Verification items for the finished model (mm, model axes). Coordinates: 2 decimals unless noted, no trailing zeros. Order: outer loops, then holes, each group sorted by start corner. A loop starts at its lowest first (then second) coordinate and runs counter-clockwise, first axis right, second up.
Q1. Cross-section at C-C, the plane y = 32. Record the boundary of the cut face in (x, z).
Q2. Depth check by flat-ended pin: P1, Ø4, axis at x = 9, z = 31, coming from the +Y side; P2, Ø1, axis at x = 8.5, z = 25.5, coming from the +Y side; P3, Ø5, axis at x = 10, y = 21.5, coming from the -Z side. Enter the tip coordinate at first touch or a pass-through.
Q3. Cross-section at B-B, the plane z = 28. Record the boundary of the cut face in (x, y).
Q4. Thickness scan on line 1 (Y direction, x = 3.25, z = 3); line 2 (Y direction, x = 1, z = 3.5); line 3 (Z direction, x = 9, y = 32.5). Record the ranges inside material, lowest first.
from build123d import *

# Parameters (mm, degrees)
BOSS_EXTRUDE1_DEPTH = 12.7
FILLET1_R           = 38.1
FILLET2_R           = 38.1


with BuildPart() as part:
    # Sketch1 → Boss-Extrude1 (new body)
    with BuildSketch(Plane(origin=(0, 0, 0), x_dir=(0, 0, -1), z_dir=(1, 0, 0))):
        Polygon((0, 0), (0, 50.8), (-50.8, 50.8), (-50.8, 38.1), (-12.7, 38.1), (-12.7, 0), align=None)
    extrude(amount=BOSS_EXTRUDE1_DEPTH)

    # Fillet1
    fillet1_edges = [part.edges().sort_by_distance(p)[0] for p in [
        (6.35, 38.1, 12.7),
    ]]
    fillet(fillet1_edges, radius=FILLET1_R - 0.0001)  # a hair under: the kernel refuses the full size

    # Fillet2
    fillet2_edges = [part.edges().sort_by_distance(p)[0] for p in [
        (6.35, 50.8, 0),
    ]]
    fillet(fillet2_edges, radius=FILLET2_R)


solid = part.part
Check values:
1. outline: (0, 5.25) - (12.7, 5.25) - (12.7, 30.12) - (0, 30.12) - close
2. P1: stops at y = 50.46
2. P2: stops at y = 48.83
2. P3: stops at z = 0.52
3. outline: (0, 30.52) - (12.7, 30.52) - (12.7, 49.44) - (0, 49.44) - close
4. line 1: y = 0 to 27.52
4. line 2: y = 0 to 28.65
4. line 3: z = 5.55 to 30.92
